Verification items for the finished model (mm, model axes). Face numbers are marked on the shaded views. A direction names the side the tool comes from. Round coordinates to 2 decimals unless told otherwise and drop trailing zeros. Loops run counter-clockwise (first coordinate to the right, second up) from the corner with the lowest first, then second, coordinate; pieces in that order, holes last. Notation, with made-up numbers: (39, -12) -> (86, -12) arc R34 cw to (86, 19) -> close; hole circle Ø11 at (51.5, -5). An arc over 180 degrees is marked (long way). Write item = value, one per line. Start each with the question number.
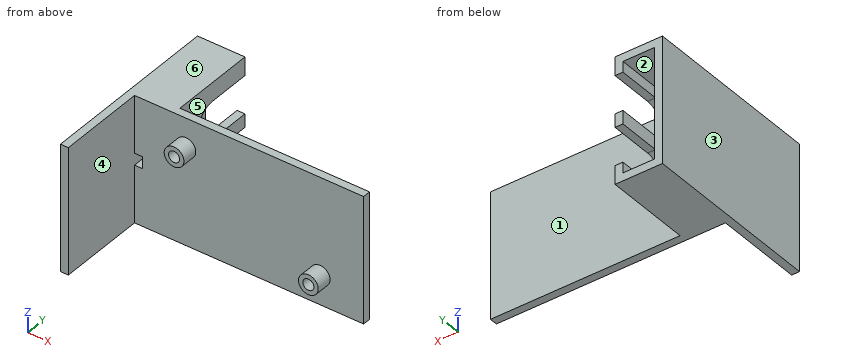
Autodesk Inventor part; units mm, degrees
ref_plane "YZ Plane" through (0, 0, 0) normal (1, 0, 0) x (0, 1, 0)
ref_plane "XZ Plane" through (0, 0, 0) normal (0, 1, 0) x (-1, 0, 0)
ref_plane "XY Plane" through (0, 0, 0) normal (0, 0, 1) x (1, 0, 0)
sketch "Sketch2" plane through (0, 0, 0) normal (1, 0, 0) x (0, 1, 0)
  line L0 (11, -16) -> (-11, -16)
  line L1 (-11, -16) -> (-11, 16)
  line L2 (-11, 16) -> (11, 16)
  line L3 (11, 16) -> (11, -16)
  line L4 (11, -16) -> (-11, 16) construction
  line L5 (-11, -16) -> (11, 16) construction
  circle A0 centre (0, -6.5) radius 4.8
  circle A1 centre (0, 6.5) radius 4.8
  line L6 (0, 6.5) -> (0, 0)
  point P0 (0, 0)
  dimension "d8" = 22
  dimension "d9" = 32
  dimension "d14" = 9.6
  dimension "d15" = 13
  dimension "d23" = 6.5
  dimension "d24" = 9.6
  dimension "d25" = 13
extrude "Extrusion2" add sketch "Sketch2" against normal blind 10
shell "Shell1" thickness 2 removed faces 3 at (-10, 8.8868, -1.7838) at (-6.6667, 4.7378, -7.27) at (-6.6667, 4.7378, 5.73)
sketch "Sketch4" plane through (0, 0, 0) normal (0, 1, 0) x (-1, 0, 0)
  line L0 (2, -14) -> (2, 14)
  line L1 (2, 0) -> (4.75, 0) construction
  line L2 (4.75, -11.3497) -> (6.75, -11.3497)
  line L3 (6.75, -11.3497) -> (6.75, 11.3497)
  line L4 (6.75, 11.3497) -> (4.75, 11.3497)
  line L5 (4.75, 11.3497) -> (4.75, -11.3497)
  point P0 (0, 0)
  dimension "d19" = 2.75
  dimension "d20" = 2
extrude "Extrusion4" [suppressed]
sketch "Sketch5" plane through (0, -11, -16) normal (0, -1, 0) x (1, 0, 0)
  line L0 (-10, 2) -> (-10, 30)
  line L1 (-8, 17.5) -> (-10, 17.5)
  line L2 (-10, 17.5) -> (-10, 14.5)
  line L3 (-10, 14.5) -> (-8, 14.5)
  line L4 (-8, 14.5) -> (-8, 17.5)
  line L5 (-8, 17.5) -> (-10, 14.5) construction
  line L6 (-10, 17.5) -> (-8, 14.5) construction
  line L7 (-10, 0) -> (-10, 32)
  point P0 (0, 16)
  dimension "d27" = 3
  dimension "d30" = 2
extrude "Extrusion5" cut sketch "Sketch5" against normal blind 2
sketch "Sketch6" plane through (-2, -9, 14) normal (-1, 0, 0) x (0, 0, 1)
  line L0 (0, 18) -> (0, 0)
  line L1 (-28, 16) -> (0, 16)
  line L2 (0, 16) -> (0, 2)
  line L3 (0, 2) -> (-28, 2)
  line L4 (-28, 2) -> (-28, 16)
  line L5 (-28, 16) -> (0, 2) construction
  line L6 (0, 16) -> (-28, 2) construction
  line L7 (-28, 18) -> (0, 18)
  line L8 (0, 18) -> (0, 0)
  line L9 (0, 0) -> (-28, 0)
  line L10 (-28, 0) -> (-28, 18)
  line L11 (-28, 18) -> (0, 0) construction
  line L12 (0, 18) -> (-28, 0) construction
  point P0 (-14, 9)
  dimension "d31" = 14
extrude "Extrusion6" add sketch "Sketch6" along normal blind 2.75 contours L0 L1 L10 L7 | L0 L9 L10 L3
sketch "Sketch7" plane through (0, -11, -16) normal (0, -1, 0) x (1, 0, 0)
  circle A0 centre (37, 7.4) radius 2.5
  circle A1 centre (3, 24.6) radius 2.5
  line L0 (-10, 14.5) -> (-10, 0)
  line L1 (-10, 0) -> (48, 0)
  line L2 (48, 0) -> (48, 32)
  line L3 (48, 32) -> (-10, 32)
  line L4 (-10, 32) -> (-10, 17.5)
  line L5 (-10, 17.5) -> (-8, 17.5)
  line L6 (-8, 17.5) -> (-8, 14.5)
  line L7 (-8, 14.5) -> (-10, 14.5)
  line L8 (-6.75, 4.6503) -> (-6.75, 27.3497)
  line L9 (-6.75, 27.3497) -> (-4.75, 27.3497)
  line L10 (-4.75, 27.3497) -> (-4.75, 4.6503)
  line L11 (-4.75, 4.6503) -> (-6.75, 4.6503)
  line L12 (-10, 0) -> (-10, 32)
  point P0 (0, 16)
extrude "Extrusion7" add sketch "Sketch7" along normal blind 2 contours A0 | A1 | L7 L6 L5 L4 L3 L2 L1 L0 | L8 L9 L10 L11
sketch "Sketch8" plane through (-10, 0, 0) normal (-1, 0, 0) x (0, 0, 1)
  line L0 (16, 11) -> (-16, 11)
  line L1 (-16, 11) -> (-16, -35.4)
  line L2 (16, -35.4) -> (-16, -35.4)
  line L3 (16, 11) -> (16, -35.4)
  point P0 (0, 0)
extrude "Extrusion8" add sketch "Sketch8" along normal blind 2
sketch "Sketch9" plane through (0, -13, -16) normal (0, -1, 0) x (1, 0, 0)
  circle A0 centre (37, 7.4) radius 1.4
  circle A1 centre (37, 7.4) radius 2.5
  circle A2 centre (3, 24.6) radius 1.4
  circle A3 centre (3, 24.6) radius 2.5
  point P0 (0, 16)
extrude "Extrusion9" add sketch "Sketch9" along normal blind 4
sketch "Sketch10" plane through (0, 0, 0) normal (1, 0, 0) x (0, 0, -1)
  line L0 (-16, 11) -> (-16, -11)
  line L1 (-16, -11) -> (16, -11)
  line L2 (16, -11) -> (16, 11)
  line L3 (16, 11) -> (-16, 11)
  circle A0 centre (-6.5, 0) radius 4.8
  circle A1 centre (6.5, 0) radius 4.8
  line L4 (16, -11) -> (16, 11)
  line L5 (16, 0) -> (-16, 0)
  line L6 (-16, -35.4) -> (-16, 11)
  line L7 (-16, 11) -> (16, 11)
  line L8 (16, 11) -> (16, 0)
  line L9 (16, 0) -> (-16, 0)
  line L10 (-16, 0) -> (-16, 11)
  point P0 (0, 0)
  point P1 (11.3, 0)
  point P2 (-11.3, 0)
  point P3 (-1.7, 0)
  point P4 (1.7, 0)
extrude "Extrusion10" cut sketch "Sketch10" against normal blind 12 contours L3 L2 L5 A1 A0 L0 | A0 L5 | L5 A1 picked at (-5.9326, 1.496) picked at (7.6976, 1.061)
sketch "Sketch11" plane through (-8, -9, 1.5) normal (0, 1, 0) x (1, 0, 0)
  line L0 (1.45, 12.6493) -> (1.45, -9.6497)
  line L1 (3.05, 12.6493) -> (1.45, 12.6493)
  line L2 (1.45, -9.6497) -> (3.05, -9.6497)
  line L3 (1.45, 12.6493) -> (3.2385, 12.6493)
  line L4 (3.2385, 12.6493) -> (3.2385, -9.6497)
  line L5 (3.2385, -9.6497) -> (1.45, -9.6497)
  line L6 (1.45, -9.6497) -> (1.45, 12.6493)
  point P0 (8, 1.5)
extrude "Extrusion11" [suppressed]
sketch "Sketch12" plane through (0, 0, -11.3) normal (0, 1, 0) x (1, 0, 0)
  line L0 (-2, -9.6) -> (0, -9.6)
  line L1 (-2, -13) -> (-2, -9.6)
  line L2 (0, -13) -> (-2, -13)
  line L3 (0, -9.6) -> (0, -13)
  line L4 (0, 0) -> (-2, 0)
  line L5 (0, 4.7) -> (0, 0)
  line L6 (-12, 4.7) -> (0, 4.7)
  line L7 (-12, -27.3) -> (-12, 4.7)
  line L8 (0, -27.3) -> (-12, -27.3)
  line L9 (0, -22.6) -> (0, -27.3)
  line L10 (-2, -22.6) -> (0, -22.6)
  line L11 (-2, -25.3) -> (-2, -22.6)
  line L12 (-10, -25.3) -> (-2, -25.3)
  line L13 (-10, 2.7) -> (-10, -25.3)
  line L14 (-2, 2.7) -> (-10, 2.7)
  line L15 (-2, 0) -> (-2, 2.7)
  point P0 (0, -11.3)
extrude "Extrusion12" add sketch "Sketch12" along normal blind 11
properties part number "snapConnector_3DPrint"
(1) Section check A-A on y = 3. Enter the section's corners in (x, z).
(2) Section check B-B on y = -6. Enter the section's corners in (x, z), then the cut area to 3 significant figures.
(3) Section check D-D on z = 8.6. Enter the section's corners in (x, y), then the cut area to 3 significant figures.
(4) Section check C-C on x = 3. Enter the section's corners in (y, z), then the cut area to 3 significant figures.
(5) Depth check by flat-ended pin: pin 1 Ø1.6 at (x, z) = (-6.5, -4.5) entering from +Y; pin 2 Ø1.5 at (x, z) = (41, 6.5) entering from +Y; pin 3 Ø2.5 at (x, z) = (3, 8.6) entering from -Y. Enter the tip coordinate at first touch or a pass-through.
(6) Scan lines: line 1 (Z direction, x = 3, y = -14.9); line 2 (X direction, y = -16, z = 8); line 3 (X direction, y = 8, z = -12). Record each from-to range of solid material in increasing order. Write a range as [from, to].
(7) Draft check along X on the marked faces 4, 5 and 6. Enter one of: +X half, -X half, draft (parallel to the pull), parting line (faces both ways), or undercut.
(8) Access from +Z, -Z, +X, -X, +Y, -Y to the whole of each face (thin tool, end or side, straight path). Record for the marked faces 1, 2 and 3.
Computed values:
q1.outline = (-12, -16) -> (0, -16) -> (0, -11.3) -> (-2, -11.3) -> (-2, -14) -> (-10, -14) -> (-10, 14) -> (-2, 14) -> (-2, 11.3) -> (0, 11.3) -> (0, 16) -> (-12, 16) -> close; (-2, -1.7) -> (0, -1.7) -> (0, 1.7) -> (-2, 1.7) -> close
q2.outline = (-12, -16) -> (0, -16) -> (0, 16) -> (-12, 16) -> close; hole (-10, -14) -> (-2, -14) -> (-2, 14) -> (-10, 14) -> close
q2.area = 160 mm²
q3.outline = (-12, -35.4) -> (-10, -35.4) -> (-10, -13) -> (0.5, -13) -> (0.5, -17) -> (1.6, -17) -> (1.6, -13) -> (4.4, -13) -> (4.4, -17) -> (5.5, -17) -> (5.5, -13) -> (48, -13) -> (48, -11) -> (0, -11) -> (0, -4.32) -> (-2, -4.32) -> (-2, -7) -> (-4.75, -7) -> (-4.75, -9) -> (-10, -9) -> (-10, 11) -> (-12, 11) -> close
q3.area = 252 mm²
q4.outline = (-17, 6.1) -> (-13, 6.1) -> (-13, -16) -> (-11, -16) -> (-11, 16) -> (-13, 16) -> (-13, 11.1) -> (-17, 11.1) -> (-17, 10) -> (-13, 10) -> (-13, 7.2) -> (-17, 7.2) -> close
q4.area = 72.8 mm²
q5.pin_1 = -9
q5.pin_2 = -11
q5.pin_3 = -13
q6.line_1 = [6.1, 7.2], [10, 11.1]
q6.line_2 = [-12, -10], [0.57, 1.74], [4.26, 5.43]
q6.line_3 = [-12, -10], [-2, 0]
q7.face_4 = undercut
q7.face_5 = +X half
q7.face_6 = draft
q8.face_1 = +Z, -Z, +X, +Y
q8.face_2 = +Y
q8.face_3 = +Z, -Z, -X, +Y, -Y
